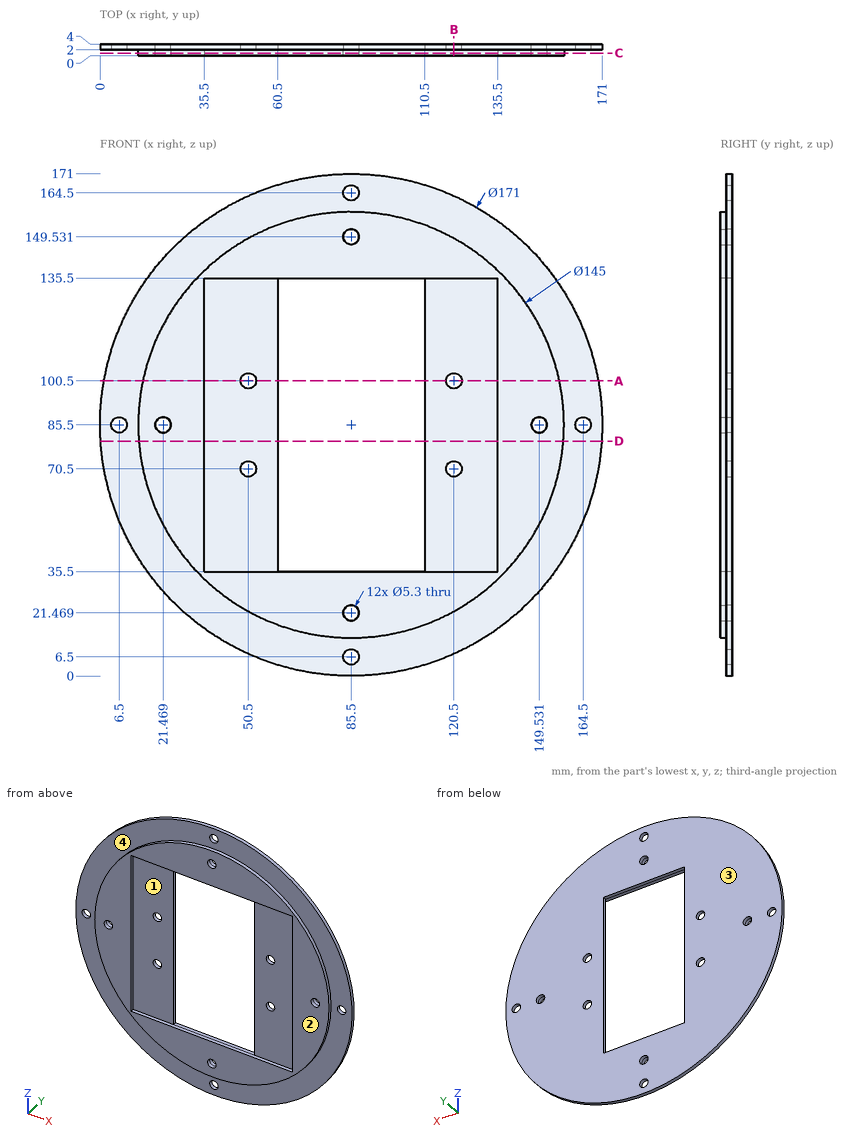
The drawing under review shows one solid part. Ordinate dimensions are in mm from its lowest x, y, z. A direction names the side the tool comes from. Round coordinates to 2 decimals unless told otherwise and drop trailing zeros. Write each loop counter-clockwise with the first axis right and the second up, starting at its lowest first coordinate (ties: lowest second). Pieces come first, ordered by that corner, then holes. Notation, with made-up numbers: (70, 16.5) -> (110, 16.5) arc R34 ccw to (110, 52.5) -> close; hole circle Ø7 at (48.25, 54.5). An arc over 180 degrees is marked (long way). One line per question, with ' | ' between items. Start each with the question number.
(1) For line 1 along Z through (x, y) = (85, 2.5); line 2 along X through (y, z) = (2.9, 85.5); line 3 along Z through (x, y) = (50, 2.9), list the stretches that pass through material, from the lowest coordinate up. Write a range as from..to.
(2) Add section C-C, the plane y = 0.9. Write out the cut boundary in (x, z).
(3) Insertion check: P1, Ø0.6, axis at y = 2.5, z = 96, coming from the +X side; P2, Ø1, axis at x = 69.5, y = 1, coming from the -Z side; P3, Ø6, axis at x = 50.5, z = 70.5, coming from the -Y side. Each pin has a flat end and moves straight along its axis. Give the tip position at first contact, or say it passes through.
(4) Add section D-D, the plane z = 80. Write out the cut boundary in (x, y).
(5) Mouldability with a two-part tool opening along Z and no side actions: class the marked faces 1 and 2 as released by +Z, released by -Z, zero draft, split by the parting line, or undercut.
(6) Add section A-A, the plane z = 100.5. Write out the cut boundary in (x, y), plus the area to 3 significant figures.
(7) Tool access review of the marked faces 3 and 4: name each direction out of +Z, -Z, +X, -X, +Y, -Y from which nothing blocks a thin tool from reaching the whole face with its end or side.
(8) Add section B-B, the plane x = 120.5. Write out the cut boundary in (y, z).
Answer list:
1) line 1: 0..3.9, 9.1..18.87, 24.07..35.5, 135.5..146.93, 152.13..161.9, 167.1..171 | line 2: 0..3.85, 9.15..18.82, 24.12..60.5, 110.5..146.88, 152.18..161.85, 167.15..171 | line 3: 7.72..67.9, 73.1..97.9, 103.1..163.28
2) outline: circle Ø145 at (85.5, 85.5); hole circle Ø5.3 at (21.47, 85.5); hole (35.5, 35.5) -> (135.5, 35.5) -> (135.5, 135.5) -> (35.5, 135.5) -> close; hole circle Ø5.3 at (85.5, 21.47); hole circle Ø5.3 at (85.5, 149.53); hole circle Ø5.3 at (149.53, 85.5)
3) P1: x = 170.39 | P2: z = 14.68 | P3: y = 2
4) outline: (0.18, 2) -> (13.21, 2) -> (13.21, 0) -> (35.5, 0) -> (35.5, 2) -> (60.5, 2) -> (60.5, 4) -> (0.18, 4) -> close; (110.5, 2) -> (135.5, 2) -> (135.5, 0) -> (157.79, 0) -> (157.79, 2) -> (170.82, 2) -> (170.82, 4) -> (110.5, 4) -> close
5) face 1: undercut | face 2: zero draft
6) outline: (1.33, 2) -> (14.57, 2) -> (14.57, 0) -> (35.5, 0) -> (35.5, 2) -> (47.85, 2) -> (47.85, 4) -> (1.33, 4) -> close; (53.15, 2) -> (60.5, 2) -> (60.5, 4) -> (53.15, 4) -> close; (110.5, 2) -> (117.85, 2) -> (117.85, 4) -> (110.5, 4) -> close; (123.15, 2) -> (135.5, 2) -> (135.5, 0) -> (156.43, 0) -> (156.43, 2) -> (169.67, 2) -> (169.67, 4) -> (123.15, 4) -> close | area: 299 mm²
7) face 3: +Z, -Z, +X, -X, +Y | face 4: -Y
8) outline: (0, 22.01) -> (2, 22.01) -> (2, 7.49) -> (4, 7.49) -> (4, 67.85) -> (2, 67.85) -> (2, 35.5) -> (0, 35.5) -> close; (0, 135.5) -> (2, 135.5) -> (2, 103.15) -> (4, 103.15) -> (4, 163.51) -> (2, 163.51) -> (2, 148.99) -> (0, 148.99) -> close; (2, 73.15) -> (4, 73.15) -> (4, 97.85) -> (2, 97.85) -> close
